```python
from build123d import *

# Parameters (mm, degrees)
SZKIC1_R                    = 17.5
SZKIC1_R_2                  = 12.6
DODANIE_WYCI_GNI_CIE1_DEPTH = 20
SZKIC2_R                    = 17.5
DODANIE_WYCI_GNI_CIE2_DEPTH = 3.5
DODANIE_WYCI_GNI_CIE3_START = -23.5
DODANIE_WYCI_GNI_CIE3_DEPTH = 23.5
SZKIC4_R                    = 3.6
SZKIC4_R_2                  = 1.6
WYTNIJ_WYCI_GNI_CIE1_DEPTH  = 41.078048855
SZKIC5_R                    = 1.75
WYTNIJ_WYCI_GNI_CIE2_DEPTH  = 52.742149163


with BuildPart() as part:
    # Szkic1 → Dodanie-wyciągnięcie1 (new body)
    with BuildSketch(Plane.XY):
        Circle(SZKIC1_R)
        Circle(SZKIC1_R_2, mode=Mode.SUBTRACT)
    extrude(amount=DODANIE_WYCI_GNI_CIE1_DEPTH)

    # Szkic2 → Dodanie-wyciągnięcie2 (add)
    with BuildSketch(Plane.XY.offset(20)):
        Circle(SZKIC2_R)
    extrude(amount=DODANIE_WYCI_GNI_CIE2_DEPTH)

    # Szkic3 → Dodanie-wyciągnięcie3 (add)
    with BuildSketch(Plane.XY.offset(23.5).offset(DODANIE_WYCI_GNI_CIE3_START)):
        with BuildLine():
            Line((-30, -12.5), (-30, -17.5))
            Line((-30, -17.5), (3e-09, -17.5))
            ThreePointArc((3e-09, -17.5), (-11.702275118, -13.011793), (-17.40200931, -1.849343661))
            Line((-17.40200931, -1.849343661), (-17.40200931, -9))
            ThreePointArc((-17.40200931, -9), (-18.427135576, -11.474873734), (-20.90200931, -12.5))
            Line((-20.90200931, -12.5), (-30, -12.5))
        make_face()
        with BuildLine():
            ThreePointArc((17.40200931, -1.849343661), (11.70227512, -13.011792998), (3e-09, -17.5))
            Line((3e-09, -17.5), (30, -17.5))
            Line((30, -17.5), (30, -12.5))
            Line((30, -12.5), (20.90200931, -12.5))
            ThreePointArc((20.90200931, -12.5), (18.427135576, -11.474873734), (17.40200931, -9))
            Line((17.40200931, -9), (17.40200931, -1.849343661))
        make_face()
    extrude(amount=DODANIE_WYCI_GNI_CIE3_DEPTH)

    # Szkic4 → Wytnij-wyciągnięcie1 (cut, through all)
    with BuildSketch(Plane(origin=(0, 0, 20), x_dir=(-1, 0, 0), z_dir=(0, 0, -1))):
        Circle(SZKIC4_R)
        with Locations((-8.8, 0)):
            Circle(SZKIC4_R_2)
        with Locations((8.8, 0)):
            Circle(SZKIC4_R_2)
    extrude(amount=-WYTNIJ_WYCI_GNI_CIE1_DEPTH, mode=Mode.SUBTRACT)

    # Szkic5 → Wytnij-wyciągnięcie2 (cut, through all)
    with BuildSketch(Plane.XZ.offset(17.5)):
        with Locations(Location((-22, 4, 0), (0, 0, 270))):
            Circle(SZKIC5_R)
        with Locations(Location((22, 4, 0), (0, 0, 231.139730474))):
            Circle(SZKIC5_R)
        with Locations(Location((22, 19.5, 0), (0, 0, 270))):
            Circle(SZKIC5_R)
        with Locations(Location((-22, 19.5, 0), (0, 0, 308.860269529))):
            Circle(SZKIC5_R)
    extrude(amount=-WYTNIJ_WYCI_GNI_CIE2_DEPTH, mode=Mode.SUBTRACT)


solid = part.part
```
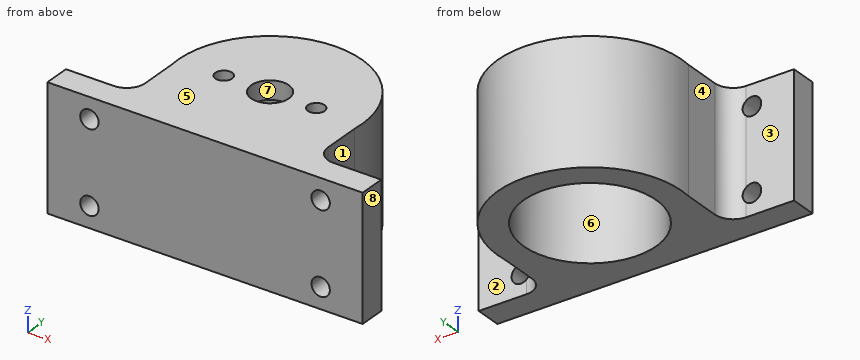
CAD build for the part. Positions are in the model's coordinates, mm. Face numbers are marked on the shaded views. A direction names the side the tool comes from. Round coordinates to 2 decimals unless told otherwise and drop trailing zeros. Loops run counter-clockwise (first coordinate to the right, second up) from the corner with the lowest first, then second, coordinate; pieces in that order, holes last. Notation, with made-up numbers: M 0.5,32 L 50.5,32 A10 cw 50.5,44 Z; hole C 88,10.25 d5. An arc over 180 degrees is marked long. Use a Markdown table: item, result. Add a question column.
(1) Drill centre lines: line 1 (X direction, y = -13.6, z = 19.5); line 2 (Z direction, x = 22, y = -14.4); line 3 (X direction, y = -0.5, z = 12). Where is each one in solid material? Low to high.
(2) Cut at C-C (x = 22). Give the cut face in (y, z).
(3) Flat gauge pins, fed straight in: pin 1 (11.5 mm diameter, centred on x = 0, y = 0, fed in from +Z); pin 2 (4.5 mm diameter, centred on x = 27.5, z = 14.5, fed in from +Y); pin 3 (5.5 mm diameter, centred on y = -6.5, z = 8.5, fed in from -X); pin 4 (4.5 mm diameter, centred on x = -22, z = 19.5, fed in from +Y) (3 decimals). Where does each tip first touch, or does it go through?
(4) Cut at D-D (z = 11.75). Give the cut face in (x, y).
(5) Cut at A-A (y = 0). Give the cut face in (x, z), and give its area (3 significant figures).
(6) Cut at B-B (z = 4.25). Give the cut face in (x, y).
(7) Pull direction X, two halves, no side cores. Call the marked faces 5, 6, 7 and 8: +X half, -X half, draft (parallel to the pull), parting line (faces both ways), or undercut.
(8) Which spindle directions (+Z, -Z, +X, -X, +Y, -Y) get a long thin tool onto all of the face, cutting with end or side? Do the marked faces 1, 2, 3 and 4. Say none if no direction does.
Geometry says:
| question | item | result |
|---|---|---|
| 1 | line 1 | x = -30 to -23.75, -20.25 to 20.25, 23.75 to 30 |
| 1 | line 2 | z = 0 to 2.25, 5.75 to 17.75, 21.25 to 23.5 |
| 1 | line 3 | x = -17.49 to -12.59, 12.59 to 17.49 |
| 2 | outline | M -17.5,0 L -12.5,0 L -12.5,2.25 L -17.5,2.25 Z; M -17.5,5.75 L -12.5,5.75 L -12.5,17.75 L -17.5,17.75 Z; M -17.5,21.25 L -12.5,21.25 L -12.5,23.5 L -17.5,23.5 Z |
| 3 | pin 1 | stops at z = 23.5 |
| 3 | pin 2 | stops at y = -12.5 |
| 3 | pin 3 | stops at x = -17.41 |
| 3 | pin 4 | stops at y = -12.305 |
| 4 | outline | M -30,-17.5 L 30,-17.5 L 30,-12.5 L 20.9,-12.5 A3.5 cw 17.4,-9 L 17.4,-1.85 A17.5 ccw long -17.4,-1.85 L -17.4,-9 A3.5 cw -20.9,-12.5 L -30,-12.5 Z; hole C 0,0 d25.2 |
| 5 | outline | M -17.5,0 L -12.6,0 L -12.6,20 L -10.4,20 L -10.4,23.5 L -17.5,23.5 Z; M -7.2,20 L -3.6,20 L -3.6,23.5 L -7.2,23.5 Z; M 3.6,20 L 7.2,20 L 7.2,23.5 L 3.6,23.5 Z; M 10.4,20 L 12.6,20 L 12.6,0 L 17.5,0 L 17.5,23.5 L 10.4,23.5 Z |
| 5 | area | 271 mm² |
| 6 | outline | M -30,-17.5 L -23.73,-17.5 L -23.73,-12.5 L -30,-12.5 Z; M -20.27,-17.5 L 20.27,-17.5 L 20.27,-12.44 A3.5 cw 17.4,-9 L 17.4,-1.85 A17.5 ccw long -17.4,-1.85 L -17.4,-9 A3.5 cw -20.27,-12.44 Z; M 23.73,-17.5 L 30,-17.5 L 30,-12.5 L 23.73,-12.5 Z; hole C 0,0 d25.2 |
| 7 | face 5 | draft |
| 7 | face 6 | undercut |
| 7 | face 7 | undercut |
| 7 | face 8 | +X half |
| 8 | face 1 | +Z, -Z, +X |
| 8 | face 2 | +Z, -Z, +X, +Y |
| 8 | face 3 | +Z, -Z, -X, +Y |
| 8 | face 4 | +Z, -Z, -X |
